from build123d import *

# Parameters (mm, degrees)
F0_R     = 5
F1_DEPTH = 7.5
F3_D     = 5.5
F4_R     = 2
F5_DEPTH = 5
F6_D     = 4.4
F6_DEPTH = 8
F6_TIP   = 1.3218933619


with BuildPart() as f1:
    # F0 (on Front) → F1 (new body, symmetric)
    with BuildSketch(Plane.XZ):
        with BuildLine():
            Line((-14.3235237483, 16), (-8.5, 0))
            Line((-8.5, 0), (35.9, 0))
            Line((35.9, 0), (35.9, 15))
            Line((35.9, 15), (7.1255015407, 15))
            Line((7.1255015407, 15), (1.7052803287, 6.1550028706))
            ThreePointArc((1.7052803287, 6.1550028706), (-0.2003761232, 5.2100629635), (-1.8793852416, 6.5159597133))
            Line((-1.8793852416, 6.5159597133), (-6.0681093439, 18.0243846007))
            Line((-6.0681093439, 18.0243846007), (-14.3235237483, 16))
        make_face()
        with Locations((10.9, 7.5)):
            Circle(F0_R, mode=Mode.SUBTRACT)
    extrude(amount=F1_DEPTH, both=True)

    # F3 (through all)
    with Locations(Plane(origin=(-7.5056888833, 0, -2.7318473412), x_dir=(0, -1, 0), z_dir=(-0.9396926208, 0, -0.3420201433))):
        with Locations((0, 13.6340155779)):
            Hole(F3_D / 2)

    # F4 (on face) → F5 (cut)
    with BuildSketch(Plane.YZ.offset(35.9)):
        with Locations((0, 2.5)):
            Circle(F4_R)
    extrude(amount=-F5_DEPTH, mode=Mode.SUBTRACT)

    # F6
    with Locations(Plane.YZ.offset(35.9)):
        with Locations((-5, 7), (5, 7)):
            Hole(F6_D / 2, depth=F6_DEPTH)
            with Locations((0, 0, -(F6_DEPTH + F6_TIP / 2))):  # 118° drill point
                Cone(0, F6_D / 2, F6_TIP, mode=Mode.SUBTRACT)


solid = f1.part
Model file for the job. Use its own axes, mm. A direction names the side the tool comes from. Give positions to 0.01 mm unless a question says otherwise; leave off trailing zeros. Order: outer loops, then holes, each group sorted by start corner. A loop starts at its lowest first (then second) coordinate and runs counter-clockwise, first axis right, second up. Notation, with made-up numbers: (-33.75, -24.75) - (-7.75, -24.75) arc R22 ccw to (-7.75, -11.75) - close; hole circle Ø8 at (-39, 62). An arc over 180 degrees is marked (long way). Write item = value, one per line. Start each with the question number.
1. Cut at C-C, the plane x = 32. List the corners of the cut face in (y, z), and give its area (3 significant figures).
2. Probe line 1 along Y through (x, z) = (30.5, 7); line 2 along Z through (x, y) = (32, -5); line 3 along Z through (x, y) = (10.9, 2.75). List the from-to ranges inside material, lowest first.
3. Drop flat-ended pins along their axis: P1, Ø2.5, axis at y = -5, z = 7, coming from the +X side; P2, Ø6, axis at y = 3.5, z = 14.5, coming from the -X side; P3, Ø4.5, axis at x = 25.5, y = -1.5, coming from the +Z side. Give the stop position or say it passes through.
4. Cut at B-B, the plane y = -0.75. List the corners of the cut face in (x, z) (3 decimals).
5. Two-plate mould, pull along X, no slides. Class faces 6 (the cylindrical face through (31.844, -6.183, 8.855)), 7 (the flat face through (35.9, 0, 7)), 8 (the flat face through (-3, -0.1, 9.6)): pulls with the +X half, pulls with the -X half, needs draft (parallel to the pull), parting line crosses it, or undercut.
6. Cut at A-A, the plane x = 10.9. List the corners of the cut face in (y, z).
7. Which spindle directions (+Z, -Z, +X, -X, +Y, -Y) get a long thin tool onto all of the face, cutting with end or side? Do faces 1 (the flat face through (16, 7.5, 9)), 2 (the cylindrical face through (33.435, -0.434, 0.548)), 3 (the flat face through (16, -7.5, 9)), 4 (the flat face through (4.453, -0.105, 10.639)), 5 (the cylindrical face through (7.666, -0.03, 14.373)). Say none if no direction does.
8. Cut at D-D, the plane y = 1.25. List the corners of the cut face in (x, z) (3 decimals), and give its area (3 significant figures).
Taken from the geometry:
q1.outline = (-7.5, 0) - (7.5, 0) - (7.5, 15) - (-7.5, 15) - close; hole circle Ø4.4 at (-5, 7); hole circle Ø4 at (0, 2.5); hole circle Ø4.4 at (5, 7)
q1.area = 182 mm²
q2.line_1 = -7.5 to -7.2, -2.8 to 2.8, 7.2 to 7.5
q2.line_2 = 0 to 4.8, 9.2 to 15
q2.line_3 = 0 to 2.5, 12.5 to 15
q3.P1 = 27.33
q3.P2 = -14.32
q3.P3 = 15
q4.outline = (-14.324, 16) - (-13.074, 12.566) - (-5.133, 15.456) - (-6.068, 18.024) - close; (-11.264, 7.594) - (-8.5, 0) - (35.9, 0) - (35.9, 0.646) - (30.9, 0.646) - (30.9, 4.354) - (35.9, 4.354) - (35.9, 15) - (9.085, 15) - (6.563, 14.082) - (1.705, 6.155) arc R2 cw to (-1.879, 6.516) - (-3.324, 10.484) - close; hole circle Ø10 at (10.9, 7.5)
q5.face_6 = needs draft
q5.face_7 = pulls with the +X half
q5.face_8 = undercut
q6.outline = (-7.5, 0) - (7.5, 0) - (7.5, 2.5) - (-7.5, 2.5) - close; (-7.5, 12.5) - (7.5, 12.5) - (7.5, 15) - (-7.5, 15) - close
q7.face_1 = +Z, -Z, +X, -X, +Y
q7.face_2 = +X
q7.face_3 = +Z, -Z, +X, -X, -Y
q7.face_4 = +Z, +Y, -Y
q7.face_5 = +Z
q8.outline = (-14.324, 16) - (-13.007, 12.382) - (-5.066, 15.272) - (-6.068, 18.024) - close; (-11.331, 7.778) - (-8.5, 0) - (35.9, 0) - (35.9, 0.939) - (30.9, 0.939) - (30.9, 4.061) - (35.9, 4.061) - (35.9, 15) - (8.511, 15) - (6.728, 14.351) - (1.705, 6.155) arc R2 cw to (-1.879, 6.516) - (-3.391, 10.668) - close; hole circle Ø10 at (10.9, 7.5)
q8.area = 518 mm²
